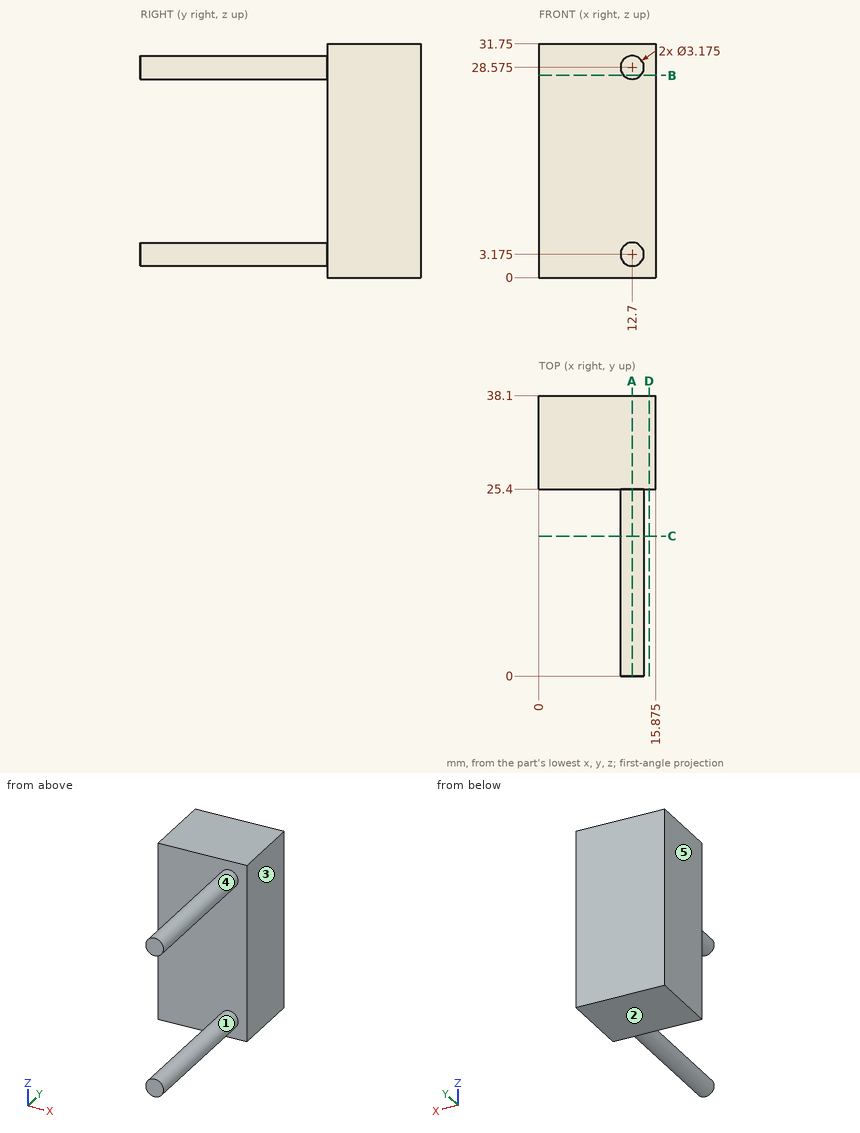
Geometry: see drawing. Coordinates: mm, zero at the bounding-box minimum. A direction names the side the tool comes from. Give positions to 0.01 mm unless a question says otherwise; leave off trailing zeros. Write each loop counter-clockwise with the first axis right and the second up, starting at its lowest first coordinate (ties: lowest second). Pieces come first, ordered by that corner, then holes. Notation, with made-up numbers: (34, 14) -> (77, 14) arc R27 ccw to (77, 44) -> close; hole circle Ø1 at (-20.5, 18.25). An arc over 180 degrees is marked (long way). Use one line per item in the form item = value. Start each with the question number.
1) Section query C-C on y = 19. Return the cut outline in (x, z) (1 decimal), then the cut area to 3 significant figures.
2) Set-up query: the marked faces 4 and 5. Return all of +Z, -Z, +X, -X, +Y, -Y with unobstructed straight access to the full face (end or side cutting, diameter ignored); none if empty.
3) Draft query along Z for the marked faces 1, 2 and 3. Return one class per face: pulls with the +Z half, pulls with the -Z half, needs draft (parallel to the pull), parting line crosses it, or undercut.
4) Section query B-B on z = 27.5. Return the cut outline in (x, y) (3 decimals), then the cut area to 3 significant figures.
5) Section query D-D on x = 15. Return the cut outline in (y, z), then the cut area to 3 significant figures.
6) Pin query (flat end, axial travel): pin 1 (5 mm diameter, centred on x = 7, z = 19.5, fed in from -Y); pin 2 (8 mm diameter, centred on x = 11, y = 31.5, fed in from -Z); pin 3 (3 mm diameter, centred on x = 13, y = 14.5, fed in from +Z). Return the tip coordinate at first contact, or that it passes through.
7) Ray query, probe 1 along Y at (x, z) = (5.25, 28.5); probe 2 along X at (y, z) = (3.5, 3); probe 3 along Z at (x, y) = (11.5, 7). Return the intervals inside material, ascending. Write a range as from..to.
8) Section query A-A on x = 12.7. Return the cut outline in (y, z), then the cut area to 3 significant figures.
Outcome:
q1.outline = circle Ø3.2 at (12.7, 3.2); circle Ø3.2 at (12.7, 28.6)
q1.area = 15.8 mm^2
q2.face_4 = -Y
q2.face_5 = +Z, -Z, -X, +Y, -Y
q3.face_1 = undercut
q3.face_2 = pulls with the -Z half
q3.face_3 = needs draft
q4.outline = (0, 25.4) -> (11.532, 25.4) -> (11.532, 0) -> (13.868, 0) -> (13.868, 25.4) -> (15.875, 25.4) -> (15.875, 38.1) -> (0, 38.1) -> close
q4.area = 261 mm^2
q5.outline = (25.4, 0) -> (38.1, 0) -> (38.1, 31.75) -> (25.4, 31.75) -> close
q5.area = 403 mm^2
q6.pin_1 = 25.4
q6.pin_2 = 0
q6.pin_3 = 30.16
q7.probe_1 = 25.4..38.1
q7.probe_2 = 11.12..14.28
q7.probe_3 = 2.14..4.21, 27.54..29.61
q8.outline = (0, 1.59) -> (25.4, 1.59) -> (25.4, 0) -> (38.1, 0) -> (38.1, 31.75) -> (25.4, 31.75) -> (25.4, 30.16) -> (0, 30.16) -> (0, 26.99) -> (25.4, 26.99) -> (25.4, 4.76) -> (0, 4.76) -> close
q8.area = 565 mm^2
